Model file for the job. Use its own axes, mm. Face numbers are marked on the shaded views. A direction names the side the tool comes from. Coordinates: 2 decimals unless noted, no trailing zeros. Order: outer loops, then holes, each group sorted by start corner. A loop starts at its lowest first (then second) coordinate and runs counter-clockwise, first axis right, second up.
Autodesk Inventor part; units mm, degrees
ref_plane "YZ Plane" through (0, 0, 0) normal (1, 0, 0) x (0, 1, 0)
ref_plane "XZ Plane" through (0, 0, 0) normal (0, 1, 0) x (-1, 0, 0)
ref_plane "XY Plane" through (0, 0, 0) normal (0, 0, 1) x (1, 0, 0)
sketch "Sketch1" plane through (0, 0, 0) normal (0, 0, 1) x (1, 0, 0)
  line L0 (0, 0) -> (4, 0)
  line L1 (4, 0) -> (4, -5)
  line L2 (4, -5) -> (0, -5)
  line L3 (0, -5) -> (0, 0)
  line L4 (0, -5) -> (-5, -5)
  line L5 (-5, -5) -> (-5, 0)
  line L6 (-5, 0) -> (0, 0)
  line L7 (0, 0) -> (0, -5)
  line L8 (-5, 0) -> (0, 0)
  line L9 (0, 0) -> (0, 3.5)
  line L10 (0, 3.5) -> (-5, 3.5)
  line L11 (-5, 3.5) -> (-5, 0)
  line L12 (-5, 3.5) -> (35, 3.5)
  line L13 (35, 3.5) -> (35, 13.5)
  line L14 (35, 13.5) -> (-5, 13.5)
  line L15 (-5, 13.5) -> (-5, 3.5)
  line L16 (-5, 1.75) -> (-15, 1.75)
  line L17 (-15, 1.75) -> (-5, 13.5)
  line L18 (-15, 1.75) -> (-5, -5)
  dimension "d0" = 4
  dimension "d1" = 5
  dimension "d2" = 5
  dimension "d3" = 3.5
  dimension "d4" = 40
  dimension "d5" = 10
  dimension "d6" = 10
extrude "Extrusion1" add sketch "Sketch1" along normal blind 15 contours L0 L1 L2 L3 | L3 L4 L5 L6 | L5 L18 L16 L11 | L10 L15 L14 L13 L12 | L16 L17 L15 L11
sketch "Sketch2" plane through (0, 0, 15) normal (0, 0, 1) x (1, 0, 0)
  line L0 (4, -5) -> (4, 0)
  line L1 (4, 0) -> (35, 0)
  line L2 (35, 0) -> (35, -5)
  line L3 (35, -5) -> (4, -5)
  line L4 (4, -5) -> (4, 0)
  line L5 (4, -5) -> (4, -25)
  line L6 (-15, 1.75) -> (-5, -5)
  line L7 (4, -25) -> (-15, 1.75)
  line L8 (-5, -5) -> (4, -5)
  line L9 (-15, 1.75) -> (-5, -5)
  line L10 (-5, -5) -> (4, -5)
  line L11 (4, -25) -> (35, -5)
  point P0 (0, 0)
  dimension "d9" = 5
  dimension "d13" = 20
extrude "Extrusion2" add sketch "Sketch2" against normal blind 5
fillet "Fillet1" radius 2 8 edges at (-15, 1.75, 5) (-15, 1.75, 12.5) (-5, 13.5, 7.5) (4, -5, 5) (35, -5, 12.5) (-5, -5, 5) (35, 13.5, 7.5) (4, -25, 12.5)
properties part number "tapeStopper_3DPrint"
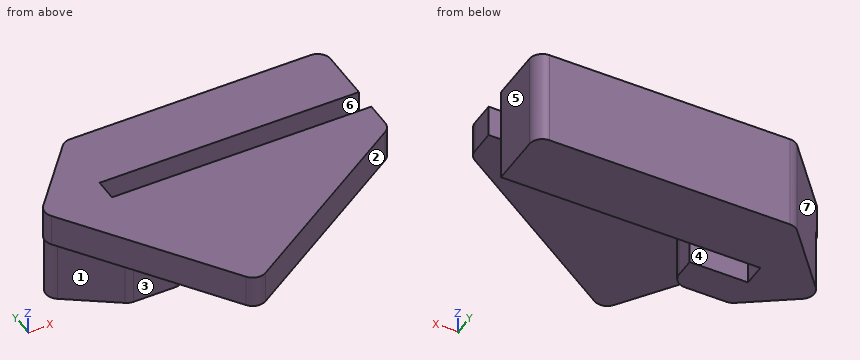
Q1. Cut at C-C, the plane x = 16. List the corners of the cut face in (y, z).
Established:
outline: (-17.26, 10) - (0, 10) - (0, 15) - (-17.26, 15) - close; (3.5, 0) - (13.5, 0) - (13.5, 15) - (3.5, 15) - close
Q2. Cut at B-B, the plane z = 12.5. List the corners of the cut face in (x, y).
Established:
outline: (-14.1, 0.48) - (2.89, -23.44) arc R2 ccw to (5.61, -23.96) - (34.08, -5.59) arc R2 ccw to (35, -3.91) - (35, 0) - (-5, 0) - (-5, 3.5) - (35, 3.5) - (35, 11.5) arc R2 ccw to (33, 13.5) - (-4.08, 13.5) arc R2 ccw to (-5.6, 12.8) - (-13.99, 2.94) arc R2 ccw to start
Q3. Which spindle directions (+Z, -Z, +X, -X, +Y, -Y) get a long thin tool onto all of the face, cutting with end or side? Do the marked faces 1, 2 and 3. Say none if no direction does.
Established:
face 1: -Z, -X, -Y
face 2: +Z, -Z, +X, -Y
face 3: -Z, +X, -X, -Y
Q4. Probe line 1 (Y direction, x = -3, z = 1.75); line 2 (Z direction, x = 2.5, y = -12); line 3 (Y direction, x = 17, z = 14). List the from-to ranges inside material, lowest first.
Established:
line 1: y = -5 to 0, 3.5 to 13.5
line 2: z = 10 to 15
line 3: y = -16.61 to 0, 3.5 to 13.5
Q5. Cut at A-A, the plane x = 8. List the corners of the cut face in (y, z).
Established:
outline: (-22.42, 10) - (0, 10) - (0, 15) - (-22.42, 15) - close; (3.5, 0) - (13.5, 0) - (13.5, 15) - (3.5, 15) - close
Q6. Mould opens along Y. For the marked faces 4, 5, 6 and 7 say: pulls with the +Y half, pulls with the -Y half, needs draft (parallel to the pull), parting line crosses it, or undercut.
Established:
face 4: undercut
face 5: needs draft
face 6: undercut
face 7: pulls with the +Y half
Q7. Cut at D-D, the plane y = 5. List the corners of the cut face in (x, z), plus the area to 3 significant figures.
Established:
outline: (-12.23, 0) - (35, 0) - (35, 15) - (-12.23, 15) - close
area: 709 mm2
Q8. Drop flat-ended pins along their axis: P1, Ø22, axis at x = 1, y = -9.5, coming from the -Z side; P2, Ø1.5, axis at y = 2, z = 8.5, coming from the -X side; P3, Ø2, axis at y = -9.5, z = 9.5, coming from the +X side; P4, Ø7, axis at x = -1, z = 4, coming from the -Y side. Give the stop position or say it passes through.
Established:
P1: stops at z = 0
P2: stops at x = -14.03
P3: stops at x = 29.37
P4: stops at y = -5
